Part print with two shaded views. Sizes in mm from the minimum x, y, z corner. Round coordinates to 2 decimals unless told otherwise and drop trailing zeros. Loops run counter-clockwise (first coordinate to the right, second up) from the corner with the lowest first, then second, coordinate; pieces in that order, holes last.
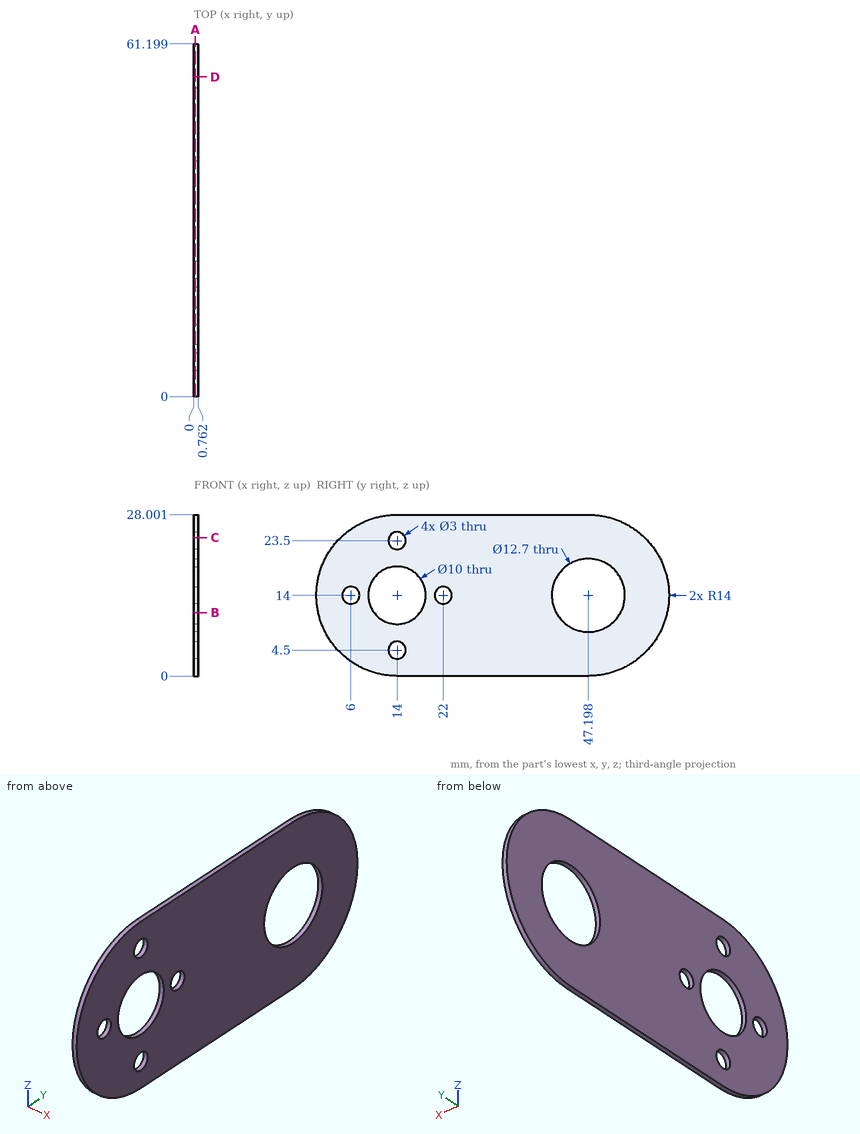
Item 1: Flat gauge pin, fed straight in: P1, Ø1.5, axis at y = 47, z = 9.5, coming from the +X side. Where does the tip first touch, or does it go through?
Verdict:
P1: passes through
Item 2: Cut at C-C (z = 24). List the corners of the cut face in (x, y) (1 decimal).
Verdict:
outline: (0, 4.2) - (0.8, 4.2) - (0.8, 12.6) - (0, 12.6) - close; (0, 15.4) - (0.8, 15.4) - (0.8, 57) - (0, 57) - close
Item 3: Cut at A-A (x = 0.25). List the corners of the cut face in (y, z).
Verdict:
outline: (14, 0) - (47.2, 0) arc R14 ccw to (47.2, 28) - (14, 28) arc R14 ccw to start; hole circle Ø3 at (6, 14); hole circle Ø10 at (14, 14); hole circle Ø3 at (14, 4.5); hole circle Ø3 at (14, 23.5); hole circle Ø3 at (22, 14); hole circle Ø12.7 at (47.2, 14)
Item 4: Cut at D-D (y = 55.5). List the corners of the cut face in (x, z) (1 decimal).
Verdict:
outline: (0, 2.7) - (0.8, 2.7) - (0.8, 25.3) - (0, 25.3) - close
Item 5: Cut at B-B (z = 11). List the corners of the cut face in (x, y) (1 decimal).
Verdict:
outline: (0, 0.3) - (0.8, 0.3) - (0.8, 10) - (0, 10) - close; (0, 18) - (0.8, 18) - (0.8, 41.6) - (0, 41.6) - close; (0, 52.8) - (0.8, 52.8) - (0.8, 60.9) - (0, 60.9) - close
Item 6: Wall check: L1, parallel to Z at x = 0.4, y = 13 (1 decimal); L2, parallel to Y at x = 0.2, z = 17 (1 decimal); L3, parallel to Z at x = 0.1, y = 6. Give the ranges that are in metal, low to high.
Verdict:
L1: z = 0 to 3.4, 5.6 to 9.1, 18.9 to 22.4, 24.6 to 28
L2: y = 0.3 to 10, 18 to 41.6, 52.8 to 60.9
L3: z = 2.51 to 12.5, 15.5 to 25.49
